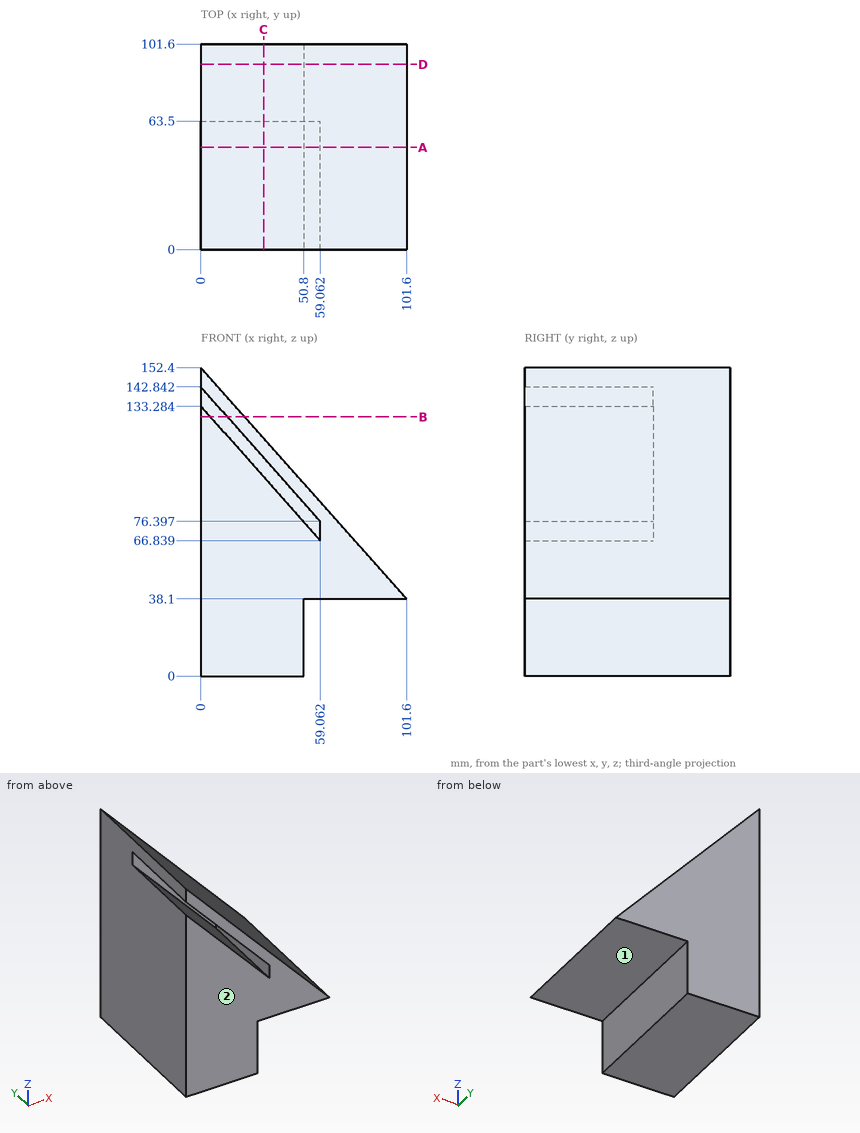
Study the drawing (mm; zero at the part's minimum x, y, z) and answer. A direction names the side the tool comes from. Round coordinates to 2 decimals unless told otherwise and drop trailing zeros. Loops run counter-clockwise (first coordinate to the right, second up) from the corner with the lowest first, then second, coordinate; pieces in that order, holes last. Notation, with made-up numbers: (56.5, 64) -> (106.5, 64) arc R21 cw to (106.5, 85) -> close; hole circle Ø9 at (-2.75, 28.5). An arc over 180 degrees is marked (long way). Use one line per item in the form item = value.
1. The part is cut by section D-D on y = 91.5. Determine the outline of the cut face in (x, z), and give its area (3 significant figures).
Answer key:
outline = (0, 0) -> (50.8, 0) -> (50.8, 38.1) -> (101.6, 38.1) -> (0, 152.4) -> close
area = 7,740 mm²
2. Find the intervals of material crossed by probe 1 along Z at (x, y) = (24, 42) (1 decimal); probe 2 along X at (y, z) = (59, 81.5) (1 decimal); probe 3 along X at (y, z) = (30, 125.5) (1 decimal), in increasing order. Write a range as [from, to].
Answer key:
probe_1 = [0, 106.3], [115.8, 125.4]
probe_2 = [0, 46], [54.5, 63]
probe_3 = [0, 6.9], [15.4, 23.9]
3. Flat-ended cylindrical pins translate along their axes: pin 1 Ø12 at (x, y) = (44.5, 42) entering from +Z; pin 2 Ø11.5 at (y, z) = (74.5, 9.5) entering from +X; pin 3 Ø1.5 at (x, y) = (44, 44) entering from +Z (1 decimal). Find the tip coordinate at first contact, or state that the pin passes through.
Answer key:
pin_1 = 109.09
pin_2 = 50.8
pin_3 = 103.7
4. The part is cut by section B-B on z = 128. Determine the outline of the cut face in (x, y).
Answer key:
outline = (0, 0) -> (4.7, 0) -> (4.7, 63.5) -> (13.19, 63.5) -> (13.19, 0) -> (21.69, 0) -> (21.69, 101.6) -> (0, 101.6) -> close
5. A tool of negligible diameter and unlimited length cuts with its end or side. For the marked faces 1 and 2, from which of +Z, -Z, +X, -X, +Y, -Y can it reach the whole face along a straight path? Write none if from no direction.
Answer key:
face_1 = -Z, +X, +Y, -Y
face_2 = +Z, -Z, +X, -X, -Y
6. The part is cut by section A-A on y = 50.5. Determine the outline of the cut face in (x, z), and give its area (3 significant figures).
Answer key:
outline = (0, 0) -> (50.8, 0) -> (50.8, 38.1) -> (101.6, 38.1) -> (0, 152.4) -> (0, 142.84) -> (59.06, 76.4) -> (59.06, 66.84) -> (0, 133.28) -> close
area = 7,180 mm²
7. The part is cut by section C-C on x = 31. Determine the outline of the cut face in (y, z) (1 decimal), and give its area (3 significant figures).
Answer key:
outline = (0, 0) -> (101.6, 0) -> (101.6, 117.5) -> (0, 117.5) -> (0, 108) -> (63.5, 108) -> (63.5, 98.4) -> (0, 98.4) -> close
area = 11,300 mm²
